```python
from build123d import *

# Parameters (mm, degrees)
F1_DEPTH  = 63.5
F0_W      = 15.1688941348
F0_H      = 12.481523478
F0_H_2    = 7.559076522
F0_H_3    = 8.5344
F2_DEPTH  = 25.4
F2_FACE_W = 50.8
F2_FACE_H = 28.575
F4_R      = 25.4
F5_R      = 25.4


with BuildPart() as f1:
    # F0 (on Front) → F1 (new body, symmetric)
    with BuildSketch(Plane.XZ):
        Polygon((28.793476522, 9.525), (-41.275, 9.525), (-41.275, -9.525), (41.275, -9.525), (41.275, 9.525), align=None)
    extrude(amount=F1_DEPTH, both=True)

    # F0 (on Front) → F2 (join, symmetric)
    with BuildSketch(Plane.XZ):
        with BuildLine():
            add(Edge.make_bspline(
                [(-41.275, 9.525), (-30.3388888889, 16.7340803864), (-19.4027777778, 23.9431607729), (-8.4666666667, 31.1522411593)],
                knots=[0, 0, 0, 0, 39.2953470054, 39.2953470054, 39.2953470054, 39.2953470054], degree=3))
            Line((-41.275, 9.525), (28.793476522, 9.525))
            Line((28.793476522, 9.525), (28.793476522, 46.0502))
            ThreePointArc((28.793476522, 46.0502), (29.3733625905, 51.7555341689), (31.0893036536, 57.2275221166))
            add(Edge.make_bspline(
                [(-8.4666666667, 31.1522411593), (4.7186567734, 39.8440014784), (17.9039802135, 48.5357617975), (31.0893036536, 57.2275221166)],
                knots=[39.2953470054, 39.2953470054, 39.2953470054, 39.2953470054, 86.6725046341, 86.6725046341, 86.6725046341, 86.6725046341], degree=3))
        make_face()
        Polygon((28.793476522, 9.525), (-41.275, 9.525), (-41.275, -9.525), (41.275, -9.525), (41.275, 9.525), align=None)
        with BuildLine():
            Line((28.793476522, 46.0502), (28.793476522, 9.525))
            Line((28.793476522, 9.525), (41.275, 9.525))
            Line((41.275, 9.525), (41.275, 46.0502))
            ThreePointArc((41.275, 46.0502), (45.9246798487, 57.2755201513), (57.15, 61.9252))
            Line((57.15, 61.9252), (57.15, 74.406723478))
            add(Edge.make_bspline(
                [(31.0893036536, 57.2275221166), (39.7762024357, 62.9539225704), (48.4631012179, 68.6803230242), (57.15, 74.406723478)],
                knots=[86.6725046341, 86.6725046341, 86.6725046341, 86.6725046341, 117.8860410162, 117.8860410162, 117.8860410162, 117.8860410162], degree=3))
            ThreePointArc((31.0893036536, 57.2275221166), (29.3733625905, 51.7555341689), (28.793476522, 46.0502))
        make_face()
        with BuildLine():
            ThreePointArc((57.15, 74.406723478), (41.543231809, 69.7255291506), (31.0893036536, 57.2275221166))
            add(Edge.make_bspline(
                [(31.0893036536, 57.2275221166), (39.7762024357, 62.9539225704), (48.4631012179, 68.6803230242), (57.15, 74.406723478)],
                knots=[86.6725046341, 86.6725046341, 86.6725046341, 86.6725046341, 117.8860410162, 117.8860410162, 117.8860410162, 117.8860410162], degree=3))
        make_face()
        with Locations((64.7344470674, 68.165961739)):
            Rectangle(F0_W, F0_H)
        with Locations((64.7344470674, 78.186261739)):
            Rectangle(F0_W, F0_H_2)
        with Locations((64.7344470674, 57.658)):
            Rectangle(F0_W, F0_H_3)
        Polygon((72.3188941348, 81.9658), (72.3188941348, 74.406723478), (72.3188941348, 61.9252), (72.3188941348, 53.3908), (107.95, 53.3908), (107.95, 81.9658), align=None)
    extrude(amount=F2_DEPTH, both=True)

    # F2_face (on face) → F3 (revolve)
    with BuildSketch(Plane(origin=(107.95, 0, 67.6783), x_dir=(0, 1, 0), z_dir=(1, 0, 0))):
        Rectangle(F2_FACE_W, F2_FACE_H)
    revolve(axis=Axis((107.95, 25.4, 67.6783), (0, 0, 1)))

    # F4
    f4_edges = [f1.edges().sort_by_distance(p)[0] for p in [
        (41.275, -63.5, 0),
        (-41.275, -63.5, 0),
    ]]
    fillet(f4_edges, radius=F4_R)

    # F5
    f5_edges = [f1.edges().sort_by_distance(p)[0] for p in [
        (-41.275, 63.5, 0),
        (41.275, 63.5, 0),
    ]]
    fillet(f5_edges, radius=F5_R)


solid = f1.part
```
Build history of the part. All positions in model axes, mm. A direction names the side the tool comes from. Give positions to 0.01 mm unless a question says otherwise; leave off trailing zeros. Loops run counter-clockwise (first coordinate to the right, second up) from the corner with the lowest first, then second, coordinate; pieces in that order, holes last.
Item 1: Slice it at B-B, the plane z = 3. List the corners of the cut face in (x, y) (3 decimals).
Answers follow:
outline: (-41.275, -38.1) arc R25.4 ccw to (-15.875, -63.5) - (15.875, -63.5) arc R25.4 ccw to (41.275, -38.1) - (41.275, 38.1) arc R25.4 ccw to (15.875, 63.5) - (-15.875, 63.5) arc R25.4 ccw to (-41.275, 38.1) - close
Item 2: Pull direction X, two halves, no side cores. Call faces 1 (the face through (41.737, -0.356, 69.852)), 2 (the face through (34.032, -55.862, 0.133)), 3 (the face through (57.15, 0, 58)): released by +X, released by -X, zero draft, split by the parting line, or undercut.
Answers follow:
face 1: released by -X
face 2: released by +X
face 3: undercut
Item 3: Flat gauge pins, fed straight in: pin 1 (7 mm diameter, centred on y = -5.5, z = 57.5, fed in from -X); pin 2 (5 mm diameter, centred on x = 14, y = -3, fed in from +Z); pin 3 (4 mm diameter, centred on y = 10, z = 78.5, fed in from -X). Where does each tip first touch, or does it go through?
Answers follow:
pin 1: stops at x = 26.19
pin 2: stops at z = 47.61
pin 3: stops at x = 57.15
Item 4: Which spindle directions (+Z, -Z, +X, -X, +Y, -Y) get a long thin tool onto all of the face, cutting with end or side? Do faces 4 (the face through (1, -45, 9.525)), 5 (the face through (19, 25.4, 35)), 6 (the face through (41.275, -1, 18)), 7 (the face through (45.8, -0.36, 57.15)). Say none if no direction does.
Answers follow:
face 4: +Z, +X, -X, -Y
face 5: +Z, -X, +Y
face 6: -Z, +X, +Y, -Y
face 7: -Z, +Y, -Y
Item 5: Slice it at C-C, the plane y = -14.5. List the corners of the cut face in (x, z) (3 decimals), and give its area (3 significant figures).
Answers follow:
outline: (-41.275, -9.525) - (41.275, -9.525) - (41.275, 46.05) arc R15.875 cw to (57.15, 61.925) - (57.15, 53.391) - (139.392, 53.391) - (139.392, 81.966) - (57.15, 81.966) - (57.15, 74.407) arc R28.357 ccw to (31.089, 57.228) - (-41.275, 9.525) - close
area: 6,440 mm2
Item 6: Slice it at D-D, the plane x = 118. List the corners of the cut face in (y, z).
Answers follow:
outline: (-24.4, 53.39) - (75.2, 53.39) - (75.2, 81.97) - (-24.4, 81.97) - close
Item 7: Slice it at A-A, the plane y = 49. List the corners of the cut face in (x, z) (3 decimals).
Answers follow:
outline: (-38.817, -9.525) - (38.817, -9.525) - (38.817, 9.525) - (-38.817, 9.525) - close; (62.965, 53.391) - (152.935, 53.391) - (152.935, 81.966) - (62.965, 81.966) - close
Item 8: Drill centre lines: line 1 (Z direction, x = 60.5, y = 1); line 2 (Y direction, x = 37, z = 51); line 3 (X direction, y = -16, z = -2) (3 decimals). Where is each one in solid material? Low to high.
Answers follow:
line 1: z = 53.39 to 81.97
line 2: y = -25.4 to 25.4
line 3: x = -41.275 to 41.275
